The model under review builds one solid part; all positions refer to its coordinate system, in mm. A direction names the side the tool comes from. Give positions to 0.01 mm unless a question says otherwise; leave off trailing zeros. Loops run counter-clockwise (first coordinate to the right, second up) from the corner with the lowest first, then second, coordinate; pieces in that order, holes last. Notation, with made-up numbers: M 15,-10.5 L 35,-10.5 A7 cw 35,-4.5 Z; hole C 21,0 d7. An arc over 180 degrees is marked long. Write item = value, one per line. Start each with the question number.
1. For faces 5 (the face through (176.647, 29, 42)), 6 (the face through (-15, -2, 0)), list the 3-axis set-ups (+Z, -Z, +X, -X, +Y, -Y) from which the entire face can be reached by the end or side of a thin tool; tool diameter is ignored.
2. Draft analysis for pull direction Z (two halves, no side actions). For faces 1 (the face through (184, 20, 63)), 2 (the face through (191.647, 6, 35)), 3 (the face through (-15, -2, 70)), 4 (the face through (184.04, 9.26, 32.62)), state which applies: pulls with the +Z half, pulls with the -Z half, needs draft (parallel to the pull), parting line crosses it, or undercut.
3. We need section B-B on z = 57. Give the boundary of the cut face in (x, y), then the cut area to 3 significant figures.
4. For pin 1 (2 mm diameter, centred on x = -1.5, z = 48.5, fed in from +Y), flat-tipped, find the tip position at first contact; note if it passes through.
5. We need section A-A on y = 20. Count the separate pieces of the cut face and the enclosed holes in it, then the cut area to 3 significant figures.
6. We need section C-C on y = 35. Give the boundary of the cut face in (x, z), then the cut area to 3 significant figures.
7. We need section D-D on z = 35. Give the boundary of the cut face in (x, y), then the cut area to 3 significant figures.
8. Wall thickness on line 1 along X through (y, z) = (9, 43); line 2 along Y through (x, z) = (-219, 57); line 3 along Y through (x, z) = (-58, 26): over which ranges is each line inside the solid? List them lowest first. Write a range as from..to.
from build123d import *

# Parameters (mm, degrees)
BOSS_EXTRUDE3_DEPTH = 70
SKETCH2_R           = 10
CUT_EXTRUDE1_DEPTH  = 408.652008458
SKETCH3_R           = 6
CUT_EXTRUDE2_DEPTH  = 408.652008458
SKETCH4_R           = 11
CUT_EXTRUDE3_DEPTH  = 408.652008458
SKETCH5_R           = 6
CUT_EXTRUDE4_DEPTH  = 408.652008458


with BuildPart() as part:
    # Sketch1 → Boss-Extrude3 (new body)
    with BuildSketch(Plane.XY):
        Polygon((-207.952872216, 0), (176.647127784, 0), (176.647127784, 40), (191.647127784, 40), (191.647127784, 0), (191.647127784, -15), (-222.952872216, -15), (-222.952872216, 0), (-222.952872216, 40), (-207.952872216, 40), align=None)
    extrude(amount=BOSS_EXTRUDE3_DEPTH)

    # Sketch2 → Cut-Extrude1 (cut, through all)
    with BuildSketch(Plane(origin=(-207.952872216, 0, 0), x_dir=(0, 0, -1), z_dir=(1, 0, 0))):
        with Locations((-35, 20)):
            Circle(SKETCH2_R)
    extrude(amount=-CUT_EXTRUDE1_DEPTH, mode=Mode.SUBTRACT)

    # Sketch3 → Cut-Extrude2 (cut, through all)
    with BuildSketch(Plane(origin=(-207.952872216, 0, 0), x_dir=(0, 0, -1), z_dir=(1, 0, 0))):
        with Locations((-13, 20)):
            Circle(SKETCH3_R)
        with Locations((-57, 20)):
            Circle(SKETCH3_R)
    extrude(amount=-CUT_EXTRUDE2_DEPTH, mode=Mode.SUBTRACT)

    # Sketch4 → Cut-Extrude3 (cut, through all)
    with BuildSketch(Plane.ZY.offset(-176.647127784)):
        with Locations((35, 20)):
            Circle(SKETCH4_R)
    extrude(amount=-CUT_EXTRUDE3_DEPTH, mode=Mode.SUBTRACT)

    # Sketch5 → Cut-Extrude4 (cut, through all)
    with BuildSketch(Plane.ZY.offset(-176.647127784)):
        with Locations(Location((57, 20, 0), (0, 0, 180))):
            Circle(SKETCH5_R)
        with Locations(Location((13, 20, 0), (0, 0, 180))):
            Circle(SKETCH5_R)
    extrude(amount=-CUT_EXTRUDE4_DEPTH, mode=Mode.SUBTRACT)


solid = part.part
Final values:
q1.face_5 = +Z, -Z, +Y
q1.face_6 = -Z, +X, -X, +Y, -Y
q2.face_1 = undercut
q2.face_2 = needs draft
q2.face_3 = pulls with the +Z half
q2.face_4 = undercut
q3.outline = M -222.95,-15 L 191.65,-15 L 191.65,14 L 176.65,14 L 176.65,0 L -207.95,0 L -207.95,14 L -222.95,14 Z; M -222.95,26 L -207.95,26 L -207.95,40 L -222.95,40 Z; M 176.65,26 L 191.65,26 L 191.65,40 L 176.65,40 Z
q3.area = 7,060 mm²
q4.pin_1 = 0
q5.separate_pieces = 8
q5.enclosed_holes = 0
q5.area = 750 mm²
q6.outline = M -222.95,0 L -207.95,0 L -207.95,70 L -222.95,70 Z; M 176.65,0 L 191.65,0 L 191.65,70 L 176.65,70 Z
q6.area = 2,100 mm²
q7.outline = M -222.95,-15 L 191.65,-15 L 191.65,9 L 176.65,9 L 176.65,0 L -207.95,0 L -207.95,10 L -222.95,10 Z; M -222.95,30 L -207.95,30 L -207.95,40 L -222.95,40 Z; M 176.65,31 L 191.65,31 L 191.65,40 L 176.65,40 Z
q7.area = 6,790 mm²
q8.line_1 = -222.95..-207.95, 176.65..191.65
q8.line_2 = -15..14, 26..40
q8.line_3 = -15..0
